Verification items for the finished model (mm, model axes). A direction names the side the tool comes from. Coordinates: 2 decimals unless noted, no trailing zeros. Write each loop counter-clockwise with the first axis right and the second up, starting at its lowest first coordinate (ties: lowest second). Pieces come first, ordered by that corner, then holes.
Autodesk Inventor part; units mm, degrees
ref_plane "YZ Plane" through (0, 0, 0) normal (1, 0, 0) x (0, 1, 0)
ref_plane "XZ Plane" through (0, 0, 0) normal (0, 1, 0) x (-1, 0, 0)
ref_plane "XY Plane" through (0, 0, 0) normal (0, 0, 1) x (1, 0, 0)
sketch "Sketch1" plane through (0, 0, 0) normal (0, 0, 1) x (1, 0, 0)
  line L0 (-22.225, -63.5) -> (-3.175, -63.5)
  line L1 (0, -63.5) -> (-25.4, -63.5)
  line L2 (-25.4, -63.5) -> (-25.4, -88.9)
  line L3 (-25.4, -88.9) -> (0, -88.9)
  line L4 (0, -88.9) -> (0, -63.5)
  line L5 (-22.225, -85.725) -> (-22.225, -66.675)
  line L6 (-22.225, -66.675) -> (-3.175, -66.675)
  line L7 (-3.175, -66.675) -> (-3.175, -85.725)
  line L8 (-3.175, -85.725) -> (-22.225, -85.725)
  point P0 (0, 0)
  dimension "d0" = 25.4
  dimension "d1" = 25.4
  dimension "d2" = 3.175
extrude "Extrusion1" add sketch "Sketch1" along normal blind 44.45
properties part number "2018 Cube Back Stop Vertical"
1. Tool access check on faces 1 (the flat face through (-25.4, -76, 22)), 2 (the flat face through (-22.225, -76, 22)). Record the directions out of +Z, -Z, +X, -X, +Y, -Y that give a thin tool (end or side, any length) a straight path to the whole face; none if there is none.
2. Material ranges on L1, parallel to Y at x = -18.25, z = 36 (3 decimals); L2, parallel to X at y = -80, z = 7 (3 decimals), recorded low to high.
3. Sectioned sample at B-B, the plane y = -67.75. Record the boundary of the cut face in (x, z) (3 decimals), and give its area (3 significant figures).
4. Sectioned sample at C-C, the plane z = 25. Record the boundary of the cut face in (x, y) (3 decimals), and give its area (3 significant figures).
5. Sectioned sample at A-A, the plane x = -12.75. Record the boundary of the cut face in (y, z) (3 decimals), and give its area (3 significant figures).
6. Draft check along Y on faces 3 (the flat face through (0, -76, 22)), 4 (the flat face through (-13, -63.5, 22)), 5 (the flat face through (-13, -66.675, 22)). Enter one of: pulls with the +Y half, pulls with the -Y half, needs draft (parallel to the pull), parting line crosses it, or undercut.
7. Gauge pin test, flat ends, axial feed: P1, Ø9.5, axis at y = -72, z = 16, coming from the +X side; P2, Ø4, axis at x = -18.5, y = -77.5, coming from the -Z side. Record the tip position at first contact, or that the pin passes through.
Outcome:
1. face 1: +Z, -Z, -X, +Y, -Y
1. face 2: +Z, -Z
2. L1: y = -88.9 to -85.725, -66.675 to -63.5
2. L2: x = -25.4 to -22.225, -3.175 to 0
3. outline: (-25.4, 0) - (-22.225, 0) - (-22.225, 44.45) - (-25.4, 44.45) - close; (-3.175, 0) - (0, 0) - (0, 44.45) - (-3.175, 44.45) - close
3. area: 282 mm2
4. outline: (-25.4, -88.9) - (0, -88.9) - (0, -63.5) - (-25.4, -63.5) - close; hole (-22.225, -85.725) - (-3.175, -85.725) - (-3.175, -66.675) - (-22.225, -66.675) - close
4. area: 282 mm2
5. outline: (-88.9, 0) - (-85.725, 0) - (-85.725, 44.45) - (-88.9, 44.45) - close; (-66.675, 0) - (-63.5, 0) - (-63.5, 44.45) - (-66.675, 44.45) - close
5. area: 282 mm2
6. face 3: needs draft
6. face 4: pulls with the +Y half
6. face 5: undercut
7. P1: stops at x = 0
7. P2: passes through
